Autodesk Inventor part; units mm, degrees
ref_plane "YZ Plane" through (0, 0, 0) normal (1, 0, 0) x (0, 1, 0)
ref_plane "XZ Plane" through (0, 0, 0) normal (0, 1, 0) x (-1, 0, 0)
ref_plane "XY Plane" through (0, 0, 0) normal (0, 0, 1) x (1, 0, 0)
sketch "Sketch1" plane through (0, 0, 0) normal (0, 0, 1) x (1, 0, 0)
  circle A0 centre (0, 0) radius 63.5 construction
  line L0 (0, 0) -> (-110.5, 0) construction
  line L1 (-110.5, 0) -> (-110.5, -80) construction
  line L2 (-110.5, -80) -> (-35.5, -80) construction
  line L3 (0, 0) -> (189.5, 0) construction
  line L4 (189.5, 0) -> (189.5, -85) construction
  line L5 (189.5, -85) -> (134.5, -85) construction
  line L6 (-93, -80) -> (-53, -80) construction
  line L7 (-53, -80) -> (-53, -85) construction
  line L8 (-53, -85) -> (-93, -85) construction
  line L9 (-93, -85) -> (-93, -80) construction
  line L10 (147, -85) -> (177, -85) construction
  line L11 (177, -85) -> (177, -90) construction
  line L12 (177, -90) -> (147, -90) construction
  line L13 (147, -90) -> (147, -85) construction
  circle A1 centre (0, 0) radius 18.5 construction
  line L14 (-35.5, -80) -> (134.5, -85) construction
  line L15 (0, 0) -> (0, -63.5) construction
  line L16 (-20.0131, 0) -> (0, -48.5) construction
  line L17 (20.0131, 0) -> (0, -48.5) construction
  line L18 (-53, -80) -> (-53, -85)
  line L19 (-53, -85) -> (-93, -85)
  line L20 (-93, -85) -> (-93, -80)
  line L21 (-93, -80) -> (-110.5, -80)
  line L22 (-110.5, -80) -> (-110.5, 0)
  line L23 (-110.5, 0) -> (-20.0131, 0) construction
  line L24 (-20.0131, 0) -> (0, -48.5) construction
  line L25 (0, -48.5) -> (20.0131, 0) construction
  line L26 (20.0131, 0) -> (189.5, 0) construction
  line L27 (189.5, 0) -> (189.5, -85) construction
  line L28 (189.5, -85) -> (177, -85)
  line L29 (177, -85) -> (177, -90)
  line L30 (177, -90) -> (147, -90)
  line L31 (147, -90) -> (147, -85)
  line L32 (147, -85) -> (79.5, -85)
  line L33 (-53, -80) -> (-35.5, -80)
  line L34 (-35.5, -80) -> (-35.5, -85)
  line L35 (-35.5, -85) -> (79.5, -85)
  line L36 (20.0131, 0) -> (70.0131, 0)
  line L37 (70.0131, 0) -> (189.5, -55)
  line L38 (189.5, -55) -> (189.5, -85)
  line L39 (0, -48.5) -> (-30, -48.5) construction
  line L40 (-30, -48.5) -> (-50.0131, 0) construction
  line L41 (12.3793, -18.5) -> (-42.3793, -18.5) construction
  line L42 (-110.5, 0) -> (-50.0131, 0)
  line L43 (-50.0131, 0) -> (-42.3793, -18.5)
  line L44 (-42.3793, -18.5) -> (12.3793, -18.5)
  line L45 (12.3793, -18.5) -> (20.0131, 0)
  dimension "d0" = 127
  dimension "d1" = 110.5
  dimension "d2" = 80
  dimension "d3" = 75
  dimension "d4" = 189.5
  dimension "d5" = 85
  dimension "d6" = 55
  dimension "d7" = 40
  dimension "d8" = 5
  dimension "d9" = 17.5
  dimension "d10" = 30
  dimension "d11" = 5
  dimension "d12" = 42.5
  dimension "d13" = 37
  dimension "d14" = 15
  dimension "d18" = 50
  dimension "d19" = 30
  dimension "d59" = 30
extrude "Extrusion1" add sketch "Sketch1" along normal blind 5
fillet "Fillet1" radius 10 4 edges at (-110.5, 0, 2.5) (20.0131, 0, 2.5) (70.0131, 0, 2.5) (189.5, -55, 2.5)
sketch "Sketch2" plane through (0, 0, 5) normal (0, 0, 1) x (1, 0, 0)
  circle A0 centre (0, 0) radius 63.5 construction
  line L0 (0, 0) -> (-110.5, 0) construction
  line L1 (-110.5, 0) -> (-110.5, -80) construction
  line L2 (0, 0) -> (189.5, 0) construction
  line L3 (189.5, 0) -> (189.5, -85) construction
  line L4 (-88, -80) -> (-63, -80) construction
  line L5 (-63, -80) -> (-63, -85) construction
  line L6 (-63, -85) -> (-88, -85) construction
  line L7 (-88, -85) -> (-88, -80) construction
  line L8 (157, -85) -> (172, -85) construction
  line L9 (172, -85) -> (172, -90) construction
  line L10 (172, -90) -> (157, -90) construction
  line L11 (157, -90) -> (157, -85) construction
  circle A1 centre (0, 0) radius 33.5 construction
  line L12 (-35.5, -80) -> (134.5, -85) construction
  line L13 (0, 0) -> (0, -63.5) construction
  line L14 (-40.8636, 0) -> (0, -58.5) construction
  line L15 (40.8636, 0) -> (0, -58.5) construction
  line L16 (-63, -80) -> (-63, -85) construction
  line L17 (-63, -85) -> (-88, -85) construction
  line L18 (-88, -85) -> (-88, -80) construction
  line L19 (-110.5, -80) -> (-110.5, 0) construction
  line L20 (-110.5, 0) -> (-40.8636, 0) construction
  line L21 (-40.8636, 0) -> (0, -58.5) construction
  line L22 (0, -58.5) -> (40.8636, 0) construction
  line L23 (40.8636, 0) -> (189.5, 0) construction
  line L24 (189.5, 0) -> (189.5, -85) construction
  line L25 (172, -85) -> (172, -90) construction
  line L26 (172, -90) -> (157, -90) construction
  line L27 (157, -90) -> (157, -85) construction
  line L28 (-35.5, -80) -> (-35.5, -85) construction
  line L29 (-35.5, -85) -> (94.5, -85) construction
  line L30 (40.8636, 0) -> (70.8636, 0) construction
  line L31 (70.8636, 0) -> (189.5, -55) construction
  line L32 (189.5, -55) -> (189.5, -85) construction
  line L33 (151, -85) -> (145, -85) construction
  line L34 (172, -85) -> (178, -85) construction
  line L35 (151, -85) -> (149, -85) construction
  line L36 (147, -85) -> (147, -70) construction
  line L37 (147, -70) -> (151, -70) construction
  line L38 (151, -70) -> (151, -85) construction
  line L39 (149, -70) -> (149, -85) construction
  line L40 (145, -78) -> (153, -78) construction
  line L41 (153, -78) -> (153, -74) construction
  line L42 (153, -74) -> (145, -74) construction
  line L43 (145, -74) -> (145, -78) construction
  line L44 (145, -78) -> (153, -74) construction
  line L45 (153, -78) -> (145, -74) construction
  line L46 (180, -85) -> (182, -85) construction
  line L47 (182, -85) -> (182, -70) construction
  line L48 (182, -70) -> (178, -70) construction
  line L49 (178, -70) -> (178, -85) construction
  line L50 (180, -70) -> (180, -85) construction
  line L51 (184, -78) -> (176, -78) construction
  line L52 (176, -78) -> (176, -74) construction
  line L53 (176, -74) -> (184, -74) construction
  line L54 (184, -74) -> (184, -78) construction
  line L55 (184, -78) -> (176, -74) construction
  line L56 (176, -78) -> (184, -74) construction
  line L57 (147, -85) -> (147, -78) construction
  line L58 (147, -85) -> (147, -78) construction
  line L59 (147, -78) -> (145, -78) construction
  line L60 (145, -78) -> (145, -74) construction
  line L61 (145, -74) -> (147, -74) construction
  line L62 (147, -74) -> (147, -70) construction
  line L63 (147, -70) -> (151, -70) construction
  line L64 (151, -70) -> (151, -74) construction
  line L65 (151, -74) -> (153, -74) construction
  line L66 (153, -74) -> (153, -78) construction
  line L67 (153, -78) -> (151, -78) construction
  line L68 (151, -78) -> (151, -85) construction
  line L69 (147, -85) -> (134.5, -85) construction
  line L70 (157, -85) -> (151, -85) construction
  line L71 (147, -85) -> (94.5, -85) construction
  line L72 (178, -85) -> (178, -78) construction
  line L73 (178, -78) -> (176, -78) construction
  line L74 (176, -78) -> (176, -74) construction
  line L75 (176, -74) -> (178, -74) construction
  line L76 (178, -74) -> (178, -70) construction
  line L77 (178, -70) -> (182, -70) construction
  line L78 (182, -70) -> (182, -74) construction
  line L79 (182, -74) -> (184, -74) construction
  line L80 (184, -74) -> (184, -78) construction
  line L81 (184, -78) -> (182, -78) construction
  line L82 (182, -78) -> (182, -85) construction
  line L83 (189.5, -85) -> (180, -85) construction
  line L84 (178, -85) -> (149, -85) construction
  line L85 (189.5, -85) -> (182, -85) construction
  line L86 (178, -85) -> (172, -85) construction
  line L87 (-98, -80) -> (-98, -65) construction
  line L88 (-98, -65) -> (-94, -65) construction
  line L89 (-94, -65) -> (-94, -80) construction
  line L90 (-55, -80) -> (-53, -80) construction
  line L91 (-53, -80) -> (-53, -65) construction
  line L92 (-53, -65) -> (-57, -65) construction
  line L93 (-57, -65) -> (-57, -80) construction
  line L94 (-96, -65) -> (-96, -80) construction
  line L95 (-55, -65) -> (-55, -80) construction
  line L96 (-100, -73) -> (-92, -73) construction
  line L97 (-92, -73) -> (-92, -69) construction
  line L98 (-92, -69) -> (-100, -69) construction
  line L99 (-100, -69) -> (-100, -73) construction
  line L100 (-100, -73) -> (-92, -69) construction
  line L101 (-92, -73) -> (-100, -69) construction
  line L102 (-51, -73) -> (-59, -73) construction
  line L103 (-59, -73) -> (-59, -69) construction
  line L104 (-59, -69) -> (-51, -69) construction
  line L105 (-51, -69) -> (-51, -73) construction
  line L106 (-51, -73) -> (-59, -69) construction
  line L107 (-59, -73) -> (-51, -69) construction
  line L108 (-98, -80) -> (-98, -73) construction
  line L109 (-98, -73) -> (-100, -73) construction
  line L110 (-100, -73) -> (-100, -69) construction
  line L111 (-100, -69) -> (-98, -69) construction
  line L112 (-98, -69) -> (-98, -65) construction
  line L113 (-98, -65) -> (-94, -65) construction
  line L114 (-94, -65) -> (-94, -69) construction
  line L115 (-94, -69) -> (-92, -69) construction
  line L116 (-92, -69) -> (-92, -73) construction
  line L117 (-92, -73) -> (-94, -73) construction
  line L118 (-94, -73) -> (-94, -80) construction
  line L119 (-88, -80) -> (-94, -80) construction
  line L120 (-98, -80) -> (-110.5, -80) construction
  line L121 (-57, -80) -> (-57, -73) construction
  line L122 (-57, -73) -> (-59, -73) construction
  line L123 (-59, -73) -> (-59, -69) construction
  line L124 (-59, -69) -> (-57, -69) construction
  line L125 (-57, -69) -> (-57, -65) construction
  line L126 (-57, -65) -> (-53, -65) construction
  line L127 (-53, -65) -> (-53, -69) construction
  line L128 (-53, -69) -> (-51, -69) construction
  line L129 (-51, -69) -> (-51, -73) construction
  line L130 (-51, -73) -> (-53, -73) construction
  line L131 (-53, -73) -> (-53, -80) construction
  line L132 (-110.5, -80) -> (-57, -80) construction
  line L133 (-55, -80) -> (-35.5, -80) construction
  line L134 (-63, -80) -> (-57, -80) construction
  line L135 (-53, -80) -> (-35.5, -80) construction
  line L136 (-88, -85) -> (-94, -85)
  line L137 (-94, -85) -> (-94, -80)
  line L138 (-94, -80) -> (-88, -80)
  line L139 (-88, -80) -> (-88, -85)
  line L140 (-94, -80) -> (-98, -80)
  line L141 (-98, -80) -> (-98, -73)
  line L142 (-98, -73) -> (-100, -73)
  line L143 (-100, -69) -> (-100, -73)
  line L144 (-100, -69) -> (-98, -69)
  line L145 (-98, -69) -> (-98, -65)
  line L146 (-98, -65) -> (-94, -65)
  line L147 (-94, -65) -> (-94, -69)
  line L148 (-94, -69) -> (-92, -69)
  line L149 (-92, -69) -> (-92, -73)
  line L150 (-92, -73) -> (-94, -73)
  line L151 (-94, -73) -> (-94, -80)
  line L152 (-110.5, -80) -> (-93, -80)
  line L153 (-63, -80) -> (-63, -85)
  line L154 (-63, -85) -> (-53, -85)
  line L155 (-53, -85) -> (-53, -73)
  line L156 (-53, -73) -> (-51, -73)
  line L157 (-51, -73) -> (-51, -69)
  line L158 (-51, -69) -> (-53, -69)
  line L159 (-53, -69) -> (-53, -65)
  line L160 (-53, -65) -> (-57, -65)
  line L161 (-57, -65) -> (-57, -69)
  line L162 (-57, -69) -> (-59, -69)
  line L163 (-59, -69) -> (-59, -73)
  line L164 (-59, -73) -> (-57, -73)
  line L165 (-57, -73) -> (-57, -80)
  line L166 (-57, -80) -> (-63, -80)
  line L167 (157, -85) -> (157, -90)
  line L168 (157, -90) -> (147, -90)
  line L169 (147, -90) -> (147, -78)
  line L170 (147, -78) -> (145, -78)
  line L171 (145, -78) -> (145, -74)
  line L172 (145, -74) -> (147, -74)
  line L173 (147, -74) -> (147, -70)
  line L174 (147, -70) -> (151, -70)
  line L175 (151, -70) -> (151, -74)
  line L176 (151, -74) -> (153, -74)
  line L177 (153, -74) -> (153, -78)
  line L178 (153, -78) -> (151, -78)
  line L179 (151, -78) -> (151, -85)
  line L180 (151, -85) -> (157, -85)
  line L181 (147, -90) -> (177, -90)
  line L182 (172, -90) -> (177, -90)
  line L183 (177, -90) -> (177, -85)
  line L184 (177, -85) -> (172, -85)
  line L185 (172, -85) -> (172, -90)
  line L186 (178, -85) -> (178, -78)
  line L187 (178, -78) -> (176, -78)
  line L188 (176, -78) -> (176, -74)
  line L189 (176, -74) -> (178, -74)
  line L190 (178, -74) -> (178, -70)
  line L191 (178, -70) -> (182, -70)
  line L192 (182, -70) -> (182, -74)
  line L193 (182, -74) -> (184, -74)
  line L194 (184, -74) -> (184, -78)
  line L195 (184, -78) -> (182, -78)
  line L196 (182, -78) -> (182, -85)
  line L197 (182, -85) -> (178, -85)
  point P0 (149, -76)
  point P1 (180, -76)
  point P2 (-96, -71)
  point P3 (-55, -71)
  dimension "d20" = 127
  dimension "d21" = 110.5
  dimension "d22" = 80
  dimension "d23" = 75
  dimension "d24" = 189.5
  dimension "d25" = 85
  dimension "d26" = 55
  dimension "d27" = 25
  dimension "d28" = 5
  dimension "d29" = 27.5
  dimension "d30" = 15
  dimension "d31" = 5
  dimension "d32" = 67
  dimension "d33" = 5
  dimension "d34" = 30
  dimension "d35" = 30
  dimension "d36" = 17.5
  dimension "d37" = 6
  dimension "d38" = 4
  dimension "d39" = 15
  dimension "d40" = 8
  dimension "d41" = 4
  dimension "d42" = 4
  dimension "d43" = 8
  dimension "d44" = 6
  dimension "d45" = 4
  dimension "d46" = 15
  dimension "d47" = 6
  dimension "d48" = 4
  dimension "d49" = 15
  dimension "d50" = 6
  dimension "d51" = 8
  dimension "d52" = 4
  dimension "d53" = 8
  dimension "d54" = 7
  dimension "d55" = 7
  dimension "d56" = 12.5
extrude "Extrusion2" cut sketch "Sketch2" against normal blind 5
fillet "Fillet2" radius 10 3 edges at (-50.0131, 0, 2.5) (-42.3793, -18.5, 2.5) (12.3793, -18.5, 2.5)
properties part number "Soporte_Ambu_Der"
Verification items for the finished model (mm, model axes). A direction names the side the tool comes from. Coordinates: 2 decimals unless noted, no trailing zeros. Loops run counter-clockwise (first coordinate to the right, second up) from the corner with the lowest first, then second, coordinate; pieces in that order, holes last. Notation, with made-up numbers: (63.25, 5.25) - (76.25, 5.25) arc R22 ccw to (76.25, 18.25) - close; hole circle Ø6 at (-3.75, 36). An arc over 180 degrees is marked (long way). Answer as a JSON object with one key per item and string values.
(1) Access from +Z, -Z, +X, -X, +Y, -Y to the whole of each face (thin tool, end or side, straight path). Record for faces 5 (the flat face through (-104, -80, 2)), 6 (the flat face through (47, 0, 2)), 7 (the cylindrical face through (11.18, -16.857, 2.535)), 8 (the flat face through (178, -82, 3)).
Response:
{"face 5": "+Z, -Z, -X, -Y", "face 6": "+Z, -Z, +X, -X, +Y", "face 7": "+Z, -Z, +Y", "face 8": "+Z, -Z, -Y"}
(2) Cross-section at B-B, the plane y = -36. Record the boundary of the cut face in (x, z).
Response:
{"outline": "(-110.5, 0) - (148.22, 0) - (148.22, 5) - (-110.5, 5) - close"}
(3) Cross-section at A-A, the plane x = 36. Record the boundary of the cut face in (y, z).
Response:
{"outline": "(-85, 0) - (0, 0) - (0, 5) - (-85, 5) - close"}
(4) Scan lines: line 1 along X through (y, z) = (-66, 2.4); line 2 along Y through (x, z) = (-81, 4.2); line 3 along X through (y, z) = (-5, 3.45). Record each from-to range of solid material in increasing order.
Response:
{"line 1": "x = -110.5 to -98, -94 to -57, -53 to 189.5", "line 2": "y = -85 to 0", "line 3": "x = -109.16 to -48.04, 18.04 to 80.88"}
(5) Mould release check, pull along X, two halves, no side actions. Record for faces 1 (the flat face through (175, -85, 2)), 2 (the flat face through (-44, -80, 2)), 3 (the cylindrical face through (-51.07, -1.74, 2.54)), 4 (the cylindrical face through (-107.49, -2.85, 2.54)): pulls with the +X half, pulls with the -X half, needs draft (parallel to the pull), parting line crosses it, or undercut.
Response:
{"face 1": "needs draft", "face 2": "undercut", "face 3": "undercut", "face 4": "pulls with the -X half"}
(6) Go/stop test with flat-tipped pins: pin 1 Ø1 at (x, z) = (146.5, 2.5) entering from -Y; pin 2 Ø1 at (x, z) = (-58.5, 3) entering from -Y; pin 3 Ø1.5 at (y, z) = (-83.5, 3.5) entering from -X. Record where each tip stops, or that it passes through.
Response:
{"pin 1": "stops at y = -85", "pin 2": "stops at y = -80", "pin 3": "stops at x = -88"}
